from build123d import *

# Parameters (mm, degrees)
BOSS_EXTRUDE1_DEPTH     = 6.35
CUT_EXTRUDE1_DEPTH      = 77.97632097
CUT_EXTRUDE1_DEPTH_BACK = 77.97632097
SKETCH10_R              = 25.000000038


with BuildPart() as part:
    # Sketch2 → Boss-Extrude1 (new body)
    with BuildSketch(Plane.XY):
        Polygon((13.749999995, 0), (41.249999987, 0), (41.249999987, -6.35), (54.999999982, -6.35), (54.999999982, 0), (54.999999982, 54.999999982), (0, 54.999999982), (0, 0), (0, -6.35), (13.749999995, -6.35), align=None)
    extrude(amount=BOSS_EXTRUDE1_DEPTH)

    # Sketch10 → Cut-Extrude1 (cut, two sides: drawn at the far end of the back side and taken through both)
    with BuildSketch(Plane(origin=(0, 4.380293547, -12.034757611), x_dir=(1, 0, 0), z_dir=(0, -0.3420201433256669, 0.9396926207859092)).offset(-CUT_EXTRUDE1_DEPTH_BACK)):
        with Locations((27.499999991, 53.753435198)):
            Circle(SKETCH10_R)
    extrude(amount=CUT_EXTRUDE1_DEPTH + CUT_EXTRUDE1_DEPTH_BACK, mode=Mode.SUBTRACT)


solid = part.part
CAD build for the part. Positions are in the model's coordinates, mm. A direction names the side the tool comes from. Round coordinates to 2 decimals unless told otherwise and drop trailing zeros. Order: outer loops, then holes, each group sorted by start corner. A loop starts at its lowest first (then second) coordinate and runs counter-clockwise, first axis right, second up. Notation, with made-up numbers: (75, 51.5) - (119, 51.5) arc R15 cw to (119, 65.5) - close; hole circle Ø6 at (0, 87). An arc over 180 degrees is marked (long way). Return JSON: item names as keys, results as strings.
(1) Cut at A-A (x = 49). Give the cut face in (y, z), then the cut area to 3 significant figures.
Answer key:
{"outline": "(-6.35, 0) - (43.63, 0) - (41.32, 6.35) - (-6.35, 6.35) - close", "area": "310 mm^2"}
(2) Tool access for faces 4 (the face through (27, 18, 0)), 5 (the face through (27, 0, 3)): list every direction of +Z, -Z, +X, -X, +Y, -Y with a clear straight run to the whole face (end or side of a thin tool).
Answer key:
{"face 4": "-Z, +X, -X, +Y, -Y", "face 5": "+Z, -Z, -Y"}
(3) Cut at B-B (x = 17). Give the cut face in (y, z), then the cut area to 3 significant figures.
Answer key:
{"outline": "(0, 0) - (33.06, 0) - (30.75, 6.35) - (0, 6.35) - close", "area": "203 mm^2"}
(4) Pull direction X, two halves, no side cores. Call faces 1 (the face through (0, 25, 3)), 2 (the face through (13.75, -3, 3)), 3 (the face through (1, 55, 3)): +X half, -X half, draft (parallel to the pull), parting line (faces both ways), or undercut.
Answer key:
{"face 1": "-X half", "face 2": "undercut", "face 3": "draft"}
(5) Wall check: probe 1 along X at (y, z) = (-3, 1); probe 2 along X at (y, z) = (34.5, 3.75); probe 3 along Y at (x, z) = (9.5, 4.5). Give the ranges that are in metal, low to high. Write a range as from..to.
Answer key:
{"probe 1": "x = 0..13.75, 41.25..55", "probe 2": "x = 0..12.57, 42.43..55", "probe 3": "y = -6.35..37.1"}
(6) Pin check, flat tip, straight feed: pin 1 Ø2 at (x, z) = (19.5, 5.5) entering from +Y. Stop position of the tip, or through.
Answer key:
{"pin 1": "stops at y = 30.52"}
